The listing builds one solid part. Answer for the finished solid, in the listing's coordinates (mm). A direction names the side the tool comes from. Round coordinates to 2 decimals unless told otherwise and drop trailing zeros. Write each loop counter-clockwise with the first axis right and the second up, starting at its lowest first coordinate (ties: lowest second). Pieces come first, ordered by that corner, then holes. Notation, with made-up numbers: (13.25, 73.5) - (58.25, 73.5) arc R24 cw to (58.25, 93.5) - close; hole circle Ø4 at (-9.75, 47). An arc over 180 degrees is marked (long way). Answer in a Markdown table with one row per item.
Autodesk Inventor part; units mm, degrees
ref_plane "YZ Plane" through (0, 0, 0) normal (1, 0, 0) x (0, 1, 0)
ref_plane "XZ Plane" through (0, 0, 0) normal (0, 1, 0) x (-1, 0, 0)
ref_plane "XY Plane" through (0, 0, 0) normal (0, 0, 1) x (1, 0, 0)
sketch "Skizze1" plane through (0, 0, 0) normal (0, 0, 1) x (1, 0, 0)
  circle A0 centre (0, 0) radius 3
  circle A1 centre (0, 0) radius 14.725
  dimension "d0" = 6
  dimension "d1" = 29.45
extrude "Extrusion1" add sketch "Skizze1" along normal mid plane 8
sketch "Skizze2" plane through (0, 0, 4) normal (0, 0, 1) x (1, 0, 0)
  circle A0 centre (0, 0) radius 3
  circle A1 centre (0, 0) radius 14.725
  circle A2 centre (0, 0) radius 4.85
  circle A3 centre (0, 0) radius 4.9
  circle A4 centre (0, 0) radius 7.325
  circle A5 centre (0, 0) radius 9.5
  circle A6 centre (0, 0) radius 7.45
  dimension "d4" = 9.7
  dimension "d5" = 9.8
  dimension "d6" = 14.65
  dimension "d7" = 19
  dimension "d16" = 14.9
extrude "Extrusion2" cut sketch "Skizze2" against normal blind 1.5 contours A2
extrude "Extrusion3" cut sketch "Skizze2" against normal blind 1.6 contours A4
extrude "Extrusion4" cut sketch "Skizze2" against normal blind 1.65 contours A5 | A6
extrude "Extrusion5" cut sketch "Skizze2" against normal blind 3 contours A3
extrude "Extrusion6" cut sketch "Skizze2" against normal blind 3 contours A6
sketch "Skizze4" plane through (0, 0, -4) normal (0, 0, -1) x (-1, 0, 0)
  circle A0 centre (0, 0) radius 3
  circle A1 centre (0, 0) radius 14.725
  circle A2 centre (0, 0) radius 4.9
  circle A3 centre (0, 0) radius 7.45
  circle A4 centre (0, 0) radius 7.325
  circle A5 centre (0, 0) radius 9.5
  circle A6 centre (0, 0) radius 4.85
extrude "Extrusion7" add sketch "Skizze4" along normal blind 3.2 contours A6
extrude "Extrusion8" cut sketch "Skizze4" against normal blind 3 contours A2
extrude "Extrusion9" cut sketch "Skizze4" against normal blind 0.6 contours A4
extrude "Extrusion10" cut sketch "Skizze4" against normal blind 3 contours A3
extrude "Extrusion11" cut sketch "Skizze4" against normal blind 0.6 contours A5
chamfer "Fase1" distance 3.175 distance2 3.4 1 edges at (-14.725, 0, -4)
chamfer "Fase2" distance 3.175 distance2 3.4 1 edges at (-14.725, 0, 4) measured on face at (12.7487, -1.9325, 4)
properties part number "Mauro_White_Wheel"
(1) For faces 4 (the flat face through (-2, -5, -3.4)), 5 (the flat face through (2, -5, 2.4)), determine the directions among +Z, -Z, +X, -X, +Y, -Y from which every point of the face is accessible in a straight line to the end or side of a thin tool.
Checked values:
| item | result |
|---|---|
| face 4 | -Z |
| face 5 | +Z |
(2) Section B-B (z = -5.75) is taken. Give the vertices of the cut face in (x, y), and give its area (3 significant figures).
Checked values:
| item | result |
|---|---|
| outline | circle Ø9.7 at (0, 0); hole circle Ø6 at (0, 0) |
| area | 45.6 mm2 |
(3) Section A-A (z = -1.5) is taken. Give the vertices of the cut face in (x, y) (3 decimals), and give its area (3 significant figures).
Checked values:
| item | result |
|---|---|
| outline | circle Ø27.769 at (0, 0); circle Ø14.65 at (0, 0); circle Ø9.7 at (0, 0); hole circle Ø14.9 at (0, 0); hole circle Ø9.8 at (0, 0); hole circle Ø6 at (0, 0) |
| area | 570 mm2 |
(4) Find the intervals of material crossed by line 1 (X direction, y = -1.5, z = -3.75); line 2 (Z direction, x = -4.5, y = -9.5); line 3 (Z direction, x = 6.25, y = 5.25), in increasing order.
Checked values:
| item | result |
|---|---|
| line 1 | x = -11.69 to -9.38, -4.61 to -2.6, 2.6 to 4.61, 9.38 to 11.69 |
| line 2 | z = -4 to 4 |
| line 3 | z = -3.4 to 2.35 |
(5) Flat-ended cylindrical pins translate along their axes: pin 1 (5 mm diameter, centred on x = -8, z = -5.5, fed in from -Y); pin 2 (16 mm diameter, centred on x = -1.5, y = 2.5, fed in from +Z); pin 3 (7.5 mm diameter, centred on x = 3, y = 0.5, fed in from +Z); pin 4 (6 mm diameter, centred on y = -8, z = 0.5, fed in from -X). Find the tip coordinate at first contact, or state that the pin passes through.
Checked values:
| item | result |
|---|---|
| pin 1 | stops at y = -10.13 |
| pin 2 | stops at z = 4 |
| pin 3 | stops at z = 2.5 |
| pin 4 | stops at x = -13.85 |
(6) For a pull along Y with two mould halves and no side action, classify faces 1 (the cylindrical face through (-3.192, -14.375, 0.008)), 2 (the flat face through (-3.2, 0.1, -7.2)), 3 (the flat face through (-6, -5, 2.35)) as pulls with the +Y half, pulls with the -Y half, needs draft (parallel to the pull), parting line crosses it, or undercut.
Checked values:
| item | result |
|---|---|
| face 1 | parting line crosses it |
| face 2 | needs draft |
| face 3 | undercut |
